from build123d import *

# Parameters (mm, degrees)
BOSS_EXTRUDE1_DEPTH = 914.4
SKETCH2_R           = 3.175
CUT_EXTRUDE1_DEPTH  = 914.4
SKETCH3_R           = 3.175
CUT_EXTRUDE2_DEPTH  = 916.10528356
CUT_EXTRUDE3_REACH  = 917.023
SKETCH4_R           = 3.175


with BuildPart() as part:
    # Sketch1 → Boss-Extrude1 (new body)
    with BuildSketch(Plane.XY):
        Polygon((0, 0), (0, 25.4), (25.4, 25.4), (25.4, 22.225), (3.175, 22.225), (3.175, 0), align=None)
    extrude(amount=BOSS_EXTRUDE1_DEPTH)

    # Sketch2 → Cut-Extrude1 (cut)
    with BuildSketch(Plane.ZY):
        with Locations((338.1375, 12.7)):
            Circle(SKETCH2_R)
        with Locations((576.2625, 12.7)):
            Circle(SKETCH2_R)
    extrude(amount=-CUT_EXTRUDE1_DEPTH, mode=Mode.SUBTRACT)

    # Sketch3 → Cut-Extrude2 (cut, through all)
    with BuildSketch(Plane(origin=(0, 25.4, 0), x_dir=(1, 0, 0), z_dir=(0, 1, 0))):
        with Locations(Location((12.7, -602.591710243, 0), (0, 0, 270))):
            Circle(SKETCH3_R)
        with Locations(Location((12.7, -311.808289757, 0), (0, 0, 270))):
            Circle(SKETCH3_R)
    extrude(amount=-CUT_EXTRUDE2_DEPTH, mode=Mode.SUBTRACT)

    # Sketch4 → Cut-Extrude3 (cut, up to next)
    with BuildSketch(Plane(origin=(3.175, 0, 0), x_dir=(0, 0, -1), z_dir=(1, 0, 0)), mode=Mode.PRIVATE) as cut_extrude3_sk1:
        with Locations((-901.7, 11.1125)):
            Circle(SKETCH4_R)
    cut_extrude3_tool1 = extrude(cut_extrude3_sk1.sketch, amount=-CUT_EXTRUDE3_REACH, mode=Mode.PRIVATE) & part.part
    # Sketch4 → Cut-Extrude3 (cut, up to next)
    with BuildSketch(Plane(origin=(3.175, 0, 0), x_dir=(0, 0, -1), z_dir=(1, 0, 0)), mode=Mode.PRIVATE) as cut_extrude3_sk2:
        with Locations((-12.7, 11.1125)):
            Circle(SKETCH4_R)
    cut_extrude3_tool2 = extrude(cut_extrude3_sk2.sketch, amount=-CUT_EXTRUDE3_REACH, mode=Mode.PRIVATE) & part.part
    add(cut_extrude3_tool1.solids().sort_by_distance((3.175, 11.1125, 901.7))[0], mode=Mode.SUBTRACT)
    add(cut_extrude3_tool2.solids().sort_by_distance((3.175, 11.1125, 12.7))[0], mode=Mode.SUBTRACT)


solid = part.part
For this review, take the finished solid that the model builds, in its own axes (mm). A direction names the side the tool comes from. Give positions to 0.01 mm unless a question says otherwise; leave off trailing zeros. Loops run counter-clockwise (first coordinate to the right, second up) from the corner with the lowest first, then second, coordinate; pieces in that order, holes last.
Item 1: Insertion check: pin 1 (5 mm diameter, centred on x = 14.5, z = 657, fed in from -Y) (3 decimals); pin 2 (4 mm diameter, centred on y = 12.7, z = 576.26, fed in from -X); pin 3 (12 mm diameter, centred on y = 16, z = 536.5, fed in from +X) (3 decimals). Each pin has a flat end and moves straight along its axis. Give the tip position at first contact, or say it passes through.
Item 2: Take a section at A-A, the plane z = 808. State the section outline as (x, y) points (3 decimals).
Item 3: For line 1 along Y through (x, z) = (1.3, 12.7); line 2 along Y through (x, z) = (14, 420.5) (3 decimals); line 3 along X through (y, z) = (3.25, 676.5) (3 decimals), list the stretches that pass through material, from the lowest coordinate up.
Item 4: Take a section at B-B, the plane x = 20.5. State the section outline as (y, z) points (3 decimals), and give its area (3 significant figures).
Item 5: Tool access review of faces 1 (the flat face through (14, 22.225, 451)), 2 (the flat face through (13, 25.4, 451)): name each direction out of +Z, -Z, +X, -X, +Y, -Y from which nothing blocks a thin tool from reaching the whole face with its end or side.
Calculated:
1. pin 1: stops at y = 22.225
1. pin 2: passes through
1. pin 3: stops at x = 3.175
2. outline: (0, 0) - (3.175, 0) - (3.175, 22.225) - (25.4, 22.225) - (25.4, 25.4) - (0, 25.4) - close
3. line 1: y = 0 to 7.94, 14.29 to 25.4
3. line 2: y = 22.225 to 25.4
3. line 3: x = 0 to 3.175
4. outline: (22.225, 0) - (25.4, 0) - (25.4, 914.4) - (22.225, 914.4) - close
4. area: 2,900 mm2
5. face 1: +Z, -Z, +X, -Y
5. face 2: +Z, -Z, +X, -X, +Y
